Geometry check sheet. Reference: the model listing, model coordinates, mm. Face numbers are marked on the shaded views. A direction names the side the tool comes from. Round coordinates to 2 decimals unless told otherwise and drop trailing zeros. Order: outer loops, then holes, each group sorted by start corner. A loop starts at its lowest first (then second) coordinate and runs counter-clockwise, first axis right, second up.
(1) Gauge pin test, flat end, axial feed: P1, Ø9.5, axis at y = 11, z = -22, coming from the -X side. Record the tip position at first contact, or that the pin passes through.
(2) Set-up check for the marked faces 5 and 6: record each of +Z, -Z, +X, -X, +Y, -Y from which the full face is reachable in a straight line by a thin tool's end or side.
(3) Cross-section at A-A on z = -15.5. Enter the section's corners in (x, y), and give its area (3 significant figures).
(4) Thickness scan on L1, parallel to Z at x = 10, y = 11.25; L2, parallel to Y at x = 13, z = -6; L3, parallel to X at y = 8.5, z = -33. Record the ranges inside material, lowest first.
(5) Draft check along Y on the marked faces 1, 2, 3 and 4. Enter one of: pulls with the +Y half, pulls with the -Y half, needs draft (parallel to the pull), parting line crosses it, or undercut.
(6) Cross-section at B-B on y = 4.5. Enter the section's corners in (x, z), and give its area (3 significant figures).
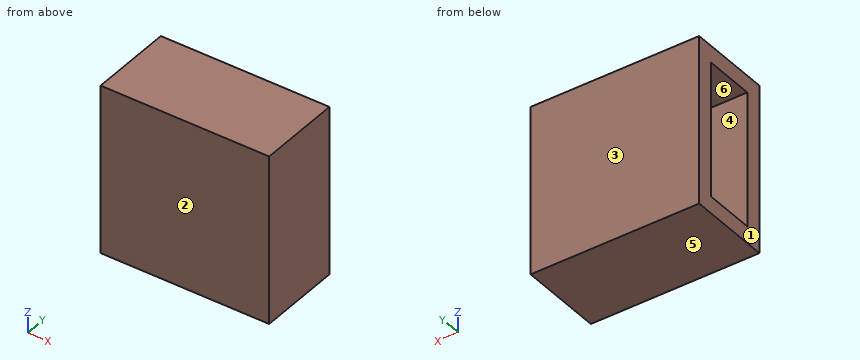
from build123d import *

# Parameters (mm, degrees)
SKETCH_1_W          = 40
SKETCH_1_H          = 40
EXTRUDE_2_DEPTH     = 20
SKETCH_2_W          = 32
SKETCH_2_H          = 12
CUT_EXTRUDE_1_DEPTH = 20


with BuildPart() as part:
    # 草图1 → 凸台-拉伸2 (new body)
    with BuildSketch(Plane(origin=(0, 0, 0), x_dir=(1, 0, 0), z_dir=(0, 1, 0))):
        with Locations((20, 20)):
            Rectangle(SKETCH_1_W, SKETCH_1_H)
    extrude(amount=EXTRUDE_2_DEPTH)

    # 草图2 → 切除-拉伸1 (cut)
    with BuildSketch(Plane.ZY):
        with Locations((-20, 10)):
            Rectangle(SKETCH_2_W, SKETCH_2_H)
    extrude(amount=-CUT_EXTRUDE_1_DEPTH, mode=Mode.SUBTRACT)


solid = part.part
Found:
1. P1: stops at x = 20
2. face 5: -Z, +X, -X, +Y, -Y
2. face 6: -X
3. outline: (0, 0) - (40, 0) - (40, 20) - (0, 20) - (0, 16) - (20, 16) - (20, 4) - (0, 4) - close
3. area: 560 mm2
4. L1: z = -40 to -36, -4 to 0
4. L2: y = 0 to 4, 16 to 20
4. L3: x = 20 to 40
5. face 1: needs draft
5. face 2: pulls with the -Y half
5. face 3: pulls with the +Y half
5. face 4: undercut
6. outline: (0, -40) - (40, -40) - (40, 0) - (0, 0) - (0, -4) - (20, -4) - (20, -36) - (0, -36) - close
6. area: 960 mm2
